```python
from build123d import *

# Parameters (mm, degrees)
SKETCH1_W               = 50.8
SKETCH1_H               = 50.8
BOSS_EXTRUDE1_DEPTH     = 6.35
SKETCH2_R               = 4.7625
CUT_EXTRUDE1_DEPTH      = 58.15
F_1_4_CLEARANCE_HOLE1_D = 6.7564
F_8_CLEARANCE_HOLE1_D   = 4.4958


with BuildPart() as part:
    # Sketch1 → Boss-Extrude1 (new body)
    with BuildSketch(Plane(origin=(0, 0, 0), x_dir=(1, 0, 0), z_dir=(0, 1, 0))):
        Rectangle(SKETCH1_W, SKETCH1_H)
    extrude(amount=BOSS_EXTRUDE1_DEPTH)

    # Sketch2 → Cut-Extrude1 (cut, through all)
    with BuildSketch(Plane.XY.offset(25.4)):
        with Locations((-9.525, -0.508)):
            Circle(SKETCH2_R)
        with Locations((9.525, -0.508)):
            Circle(SKETCH2_R)
    extrude(amount=-CUT_EXTRUDE1_DEPTH, mode=Mode.SUBTRACT)

    # 1/4 Clearance Hole1 (through all)
    with Locations(Plane(origin=(0, 6.35, 0), x_dir=(1, 0, 0), z_dir=(0, 1, 0))):
        with Locations((-20.6375, -20.6375), (-20.6375, 20.6375), (20.6375, 20.6375), (20.6375, -20.6375)):
            Hole(F_1_4_CLEARANCE_HOLE1_D / 2)

    # #8 Clearance Hole1 (through all)
    with Locations(Plane(origin=(0, 6.35, 0), x_dir=(1, 0, 0), z_dir=(0, 1, 0))):
        with Locations((0, 12.7), (0, -12.7)):
            Hole(F_8_CLEARANCE_HOLE1_D / 2)


solid = part.part
```
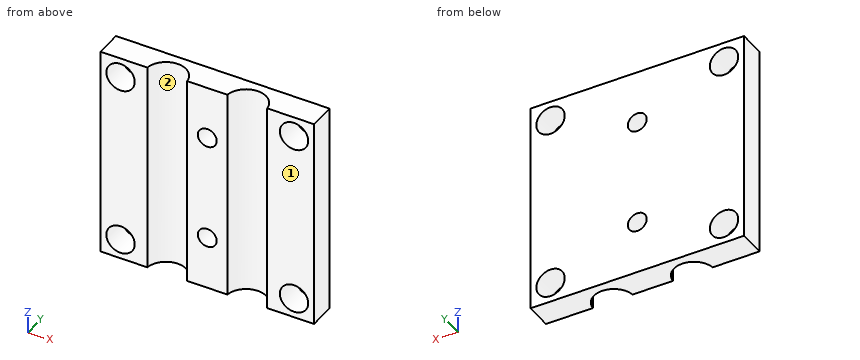
Geometry check sheet. Reference: the model listing, model coordinates, mm. Face numbers are marked on the shaded views. Give positions to 0.01 mm unless a question says otherwise; leave off trailing zeros. Order: outer loops, then holes, each group sorted by start corner. A loop starts at its lowest first (then second) coordinate and runs counter-clockwise, first axis right, second up.
1. Section check D-D, the plane y = 5.5. Enter the section's corners in (x, z).
2. Release check for a two-part mould opening along X. For the marked faces 1 and 2 record: pulls with the +X half, pulls with the -X half, needs draft (parallel to the pull), parting line crosses it, or undercut.
3. Section check C-C, the plane x = 0. Enter the section's corners in (y, z).
4. Thickness scan on L1, parallel to Z at x = 0, y = 5; L2, parallel to X at y = 2.75, z = 9; L3, parallel to Z at x = 22, y = 6.25. Record the ranges inside material, lowest first.
5. Section check A-A, the plane y = 1.25. Give the number of separate pieces and of enclosed holes in the cut face, and give its area (3 significant figures).
6. Gauge pin test, flat end, axial feed: pin 1 Ø1 at (x, z) = (14, 8) entering from -Y. Record the tip position at first contact, or that the pin passes through.
Values follow:
1. outline: (-25.4, -25.4) - (25.4, -25.4) - (25.4, 25.4) - (-25.4, 25.4) - close; hole circle Ø6.76 at (-20.64, -20.64); hole circle Ø6.76 at (-20.64, 20.64); hole circle Ø4.5 at (0, -12.7); hole circle Ø4.5 at (0, 12.7); hole circle Ø6.76 at (20.64, -20.64); hole circle Ø6.76 at (20.64, 20.64)
2. face 1: needs draft
2. face 2: undercut
3. outline: (0, -25.4) - (6.35, -25.4) - (6.35, -14.95) - (0, -14.95) - close; (0, -10.45) - (6.35, -10.45) - (6.35, 10.45) - (0, 10.45) - close; (0, 14.95) - (6.35, 14.95) - (6.35, 25.4) - (0, 25.4) - close
4. L1: z = -25.4 to -14.95, -10.45 to 10.45, 14.95 to 25.4
4. L2: x = -25.4 to -13, -6.05 to 6.05, 13 to 25.4
4. L3: z = -25.4 to -23.73, -17.55 to 17.55, 23.73 to 25.4
5. separate pieces: 3
5. enclosed holes: 6
5. area: 1,510 mm2
6. pin 1: stops at y = 0
